```python
from build123d import *

# Parameters (mm, degrees)
BASE_FLANGE1_START                     = -3
BASE_FLANGE1_OUTLINE_W                 = 110
BASE_FLANGE1_OUTLINE_H                 = 500
BASE_FLANGE1_DEPTH                     = 3
T_LE_PLI_E_SUR_AR_TE1_STRIP_W          = 13.4732
T_LE_PLI_E_SUR_AR_TE1_STRIP_H          = 3
T_LE_PLI_E_SUR_AR_TE1_STRIP_CUT_DEPTH  = 80
T_LE_PLI_E_SUR_AR_TE1_RELIEF_W         = 14.9732
T_LE_PLI_E_SUR_AR_TE1_RELIEF_H         = 1.5
T_LE_PLI_E_SUR_AR_TE1_RELIEF_CUT_DEPTH = 3
T_LE_PLI_E_SUR_AR_TE1_DEPTH            = 80
FILLET2_R                              = 3
CUT_EXTRUDE2_DEPTH                     = 552.574796719
CUT_EXTRUDE2_DEPTH_BACK                = 3
F_7_1_7_1_DIAMETER_SLOT1_D             = 7.1
F_7_1_7_1_DIAMETER_SLOT1_DEPTH         = 3
F_7_1_7_1_DIAMETER_SLOT1_TIP           = 2.133055198


# Read off the part's stored shape, not the designer's step: Base-Flange1
# Sheet-metal steps are written as plain solids
with BuildPart() as part:
    # Base-Flange1 outline → Base-Flange1 (new body)
    with BuildSketch(Plane(origin=(0, 0, 0), x_dir=(1, 0, 0), z_dir=(0, 1, 0)).offset(BASE_FLANGE1_START)):
        with Locations((59.130435799, 250)):
            Rectangle(BASE_FLANGE1_OUTLINE_W, BASE_FLANGE1_OUTLINE_H)
    extrude(amount=BASE_FLANGE1_DEPTH)

    # Tôle pliée sur arête1 strip (across the edge) → Tôle pliée sur arête1 strip cut (cut)
    with BuildSketch(Plane(origin=(19.130435799, 0, 0), x_dir=(0, 0, -1), z_dir=(1, 0, 0))):
        with Locations((-3, -1.5)):
            Rectangle(T_LE_PLI_E_SUR_AR_TE1_STRIP_W, T_LE_PLI_E_SUR_AR_TE1_STRIP_H)
    extrude(amount=T_LE_PLI_E_SUR_AR_TE1_STRIP_CUT_DEPTH, mode=Mode.SUBTRACT)

    # Tôle pliée sur arête1 relief (on the sheet) → Tôle pliée sur arête1 relief cut (cut)
    with BuildSketch(Plane(origin=(19.130435799, 0, -3.7366), x_dir=(0, 0, -1), z_dir=(0, 1, 0))):
        with Locations((-5.9866, 0.75)):
            Rectangle(T_LE_PLI_E_SUR_AR_TE1_RELIEF_W, T_LE_PLI_E_SUR_AR_TE1_RELIEF_H)
        with Locations((-5.9866, -80.75)):
            Rectangle(T_LE_PLI_E_SUR_AR_TE1_RELIEF_W, T_LE_PLI_E_SUR_AR_TE1_RELIEF_H)
    extrude(amount=-T_LE_PLI_E_SUR_AR_TE1_RELIEF_CUT_DEPTH, mode=Mode.SUBTRACT)

    # Tôle pliée sur arête1 section (across the edge) → Tôle pliée sur arête1 (add)
    with BuildSketch(Plane(origin=(19.130435799, 0, 0), x_dir=(0, 0, -1), z_dir=(1, 0, 0))):
        with BuildLine():
            Line((0, 0.7366), (0, 200))
            Line((0, 200), (3, 200))
            Line((3, 200), (3, 0.7366))
            ThreePointArc((3, 0.7366), (3.215745145, 0.215745145), (3.7366, 0))
            Line((3.7366, 0), (3.7366, -3))
            ThreePointArc((3.7366, -3), (1.094424801, -1.905575199), (0, 0.7366))
        make_face()
    extrude(amount=T_LE_PLI_E_SUR_AR_TE1_DEPTH)

    # Fillet2
    fillet2_edges = [part.edges().sort_by_distance(p)[0] for p in [
        (19.130435799, 200, -1.5),
        (99.130435799, 200, -1.5),
        (4.130435799, -1.5, -500),
        (114.130435799, -1.5, -500),
    ]]
    fillet(fillet2_edges, radius=FILLET2_R)

    # Sketch14 → Cut-Extrude2 (cut, two sides: drawn at the far end of the back side and taken through both)
    with BuildSketch(Plane.XZ.offset(3).offset(-CUT_EXTRUDE2_DEPTH_BACK)):
        with BuildLine():
            Line((1095.888112959, -26.7366), (114.130435799, -26.7366))
            Line((114.130435799, -26.7366), (108.694609025, -26.7366))
            Line((108.694609025, -26.7366), (108.694609025, -226.7366))
            Line((108.694609025, -226.7366), (114.130435799, -226.7366))
            Line((114.130435799, -226.7366), (114.130435799, -241.7366))
            Line((114.130435799, -241.7366), (73.130435799, -263.202647067))
            ThreePointArc((73.130435799, -263.202647067), (78.953729303, -305.702647067), (73.130435799, -348.202647067))
            ThreePointArc((73.130435799, -348.202647067), (88.130435799, -363.202647067), (73.130435799, -378.202647067))
            Line((73.130435799, -378.202647067), (103.130435799, -378.202647067))
            Line((103.130435799, -378.202647067), (103.130435799, -500))
            Line((103.130435799, -500), (15.130435799, -500))
            Line((15.130435799, -500), (15.130435799, -378.202647067))
            Line((15.130435799, -378.202647067), (45.130435799, -378.202647067))
            ThreePointArc((45.130435799, -378.202647067), (30.130435799, -363.202647067), (45.130435799, -348.202647067))
            ThreePointArc((45.130435799, -348.202647067), (39.307142295, -305.702647067), (45.130435799, -263.202647067))
            Line((45.130435799, -263.202647067), (4.130435799, -241.7366))
            Line((4.130435799, -241.7366), (4.130435799, -226.7366))
            Line((4.130435799, -226.7366), (9.566262574, -226.7366))
            Line((9.566262574, -226.7366), (9.566262574, -26.7366))
            Line((9.566262574, -26.7366), (4.130435799, -26.7366))
            Line((4.130435799, -26.7366), (-977.62724136, -26.7366))
            Line((-977.62724136, -26.7366), (-977.62724136, -1990.251954319))
            Line((-977.62724136, -1990.251954319), (1095.888112959, -1990.251954319))
            Line((1095.888112959, -1990.251954319), (1095.888112959, -26.7366))
        make_face()
    extrude(amount=CUT_EXTRUDE2_DEPTH + CUT_EXTRUDE2_DEPTH_BACK, mode=Mode.SUBTRACT)

    # Ø7.1 (7.1) Diameter Slot1
    with Locations(Plane(origin=(0, -3, 0), x_dir=(-1, 0, 0), z_dir=(0, -1, 0))):
        with Locations((-59.130435799, 476.35), (-89.450435799, 456.35), (-28.810435799, 456.35)):
            Hole(F_7_1_7_1_DIAMETER_SLOT1_D / 2, depth=F_7_1_7_1_DIAMETER_SLOT1_DEPTH)
            with Locations((0, 0, -(F_7_1_7_1_DIAMETER_SLOT1_DEPTH + F_7_1_7_1_DIAMETER_SLOT1_TIP / 2))):  # 118° drill point
                Cone(0, F_7_1_7_1_DIAMETER_SLOT1_D / 2, F_7_1_7_1_DIAMETER_SLOT1_TIP, mode=Mode.SUBTRACT)


solid = part.part
```
Work out the finished part from the listing and answer in its coordinate system (mm). A direction names the side the tool comes from. Coordinates: 2 decimals unless noted, no trailing zeros. Loops run counter-clockwise (first coordinate to the right, second up) from the corner with the lowest first, then second, coordinate; pieces in that order, holes last. Notation, with made-up numbers: M -35.5,-37.75 L -24.5,-37.75 A16 cw -24.5,-6.75 Z; hole C 85.25,-5.75 d3. An arc over 180 degrees is marked long. Use CSV: the item, a comma, the result in double quotes. Start each with the question number.
(1) Find section B-B, the plane z = -389. Give the vertices of the cut face in (x, y), then the cut area to 3 significant figures.
(2) Consider line 1 (X direction, y = -2.1, z = -456.35); line 2 (X direction, y = -2, z = -456); line 3 (Y direction, x = 76.5, z = -331). Determine where each line is inside the solid, lowest interval first.
(3) Given pin 1 Ø0.8 at (x, y) = (100, -1.5) entering from +Z; pin 2 Ø0.9 at (y, z) = (-1, -121.5) entering from +X; pin 3 Ø1.5 at (x, y) = (6, -1.5) entering from +Z; pin 4 Ø2.5 at (y, z) = (-1, -438.5) entering from +X, each flat-ended and moving along its own axis, determine where each tip first touches the part or whether it passes through.
(4) For faces 1 (the face through (24.92, -1.48, -252.62)), 2 (the face through (93.92, -1.48, -252.32)), determine the directions among +Z, -Z, +X, -X, +Y, -Y from which every point of the face is accessible in a straight line to the end or side of a thin tool.
(5) Find section A-A, the plane y = 98. Give the vertices of the cut face in (x, z), then the cut area to 3 significant figures.
(6) For a pull along Z with two mould halves and no side action, classify faces 3 (the face through (58, -3, -254)), 4 (the face through (59, 102, -3)), 5 (the face through (88.127, -1.479, -362.873)), 6 (the face through (59, 99, 0)) as +Z half, -Z half, draft (parallel to the pull), parting line (faces both ways), or undercut.
Recorded:
1,outline,"M 15.13,-3 L 103.13,-3 L 103.13,0 L 15.13,0 Z"
1,area,"264 mm^2"
2,line 1,"x = 15.13 to 25.26, 32.36 to 85.9, 93 to 103.13"
2,line 2,"x = 15.13 to 25.28, 32.34 to 85.92, 92.98 to 103.13"
2,line 3,"y = -3 to 0"
3,pin 1,"stops at z = -5.24"
3,pin 2,"stops at x = 108.69"
3,pin 3,"stops at z = 0"
3,pin 4,"stops at x = 103.13"
4,face 1,"-X, +Y, -Y"
4,face 2,"+X, +Y, -Y"
5,outline,"M 19.13,-3 L 99.13,-3 L 99.13,0 L 19.13,0 Z"
5,area,"240 mm^2"
6,face 3,"draft"
6,face 4,"-Z half"
6,face 5,"undercut"
6,face 6,"+Z half"
